For this review, take the finished solid that the model builds, in its own axes (mm). Round coordinates to 2 decimals unless told otherwise and drop trailing zeros. Order: outer loops, then holes, each group sorted by start corner. A loop starts at its lowest first (then second) coordinate and runs counter-clockwise, first axis right, second up.
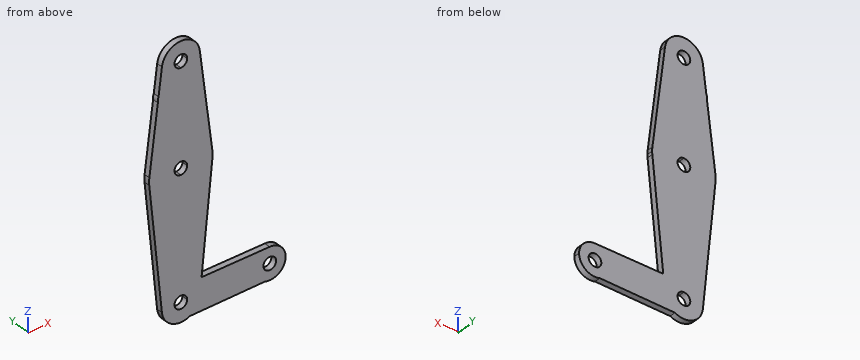
```python
from build123d import *

# Parameters (mm, degrees)
F1_DEPTH = 3.048


with BuildPart() as f1:
    # F0 (on Front) → F1 (new body)
    with BuildSketch(Plane.XZ):
        with BuildLine():
            ThreePointArc((-9.4502929642, 115.490625), (-7.14375, 107.9998046905), (0, 104.775))
            ThreePointArc((0, 104.775), (6.7351920908, 107.5648079092), (9.525, 114.3))
            ThreePointArc((9.525, 114.3), (9.5063048942, 114.896483242), (9.4502929642, 115.490625))
            ThreePointArc((9.4502929642, 115.490625), (0, 123.825), (-9.4502929642, 115.490625))
        make_face()
        with BuildLine():
            ThreePointArc((3.175, 114.3), (2.2450640303, 112.0549359697), (0, 111.125))
            ThreePointArc((0, 111.125), (-2.2450640303, 116.5450640303), (3.175, 114.3))
        make_face(mode=Mode.SUBTRACT)
        with BuildLine():
            ThreePointArc((9.525, 114.3), (6.7351920908, 107.5648079092), (0, 104.775))
            Line((0, 104.775), (0, 79.375))
            ThreePointArc((0, 79.375), (10.5003255158, 75.40625), (15.7504882737, 65.484375))
            Line((15.7504882737, 65.484375), (9.4502929642, 115.490625))
            ThreePointArc((9.4502929642, 115.490625), (9.5063048942, 114.896483242), (9.525, 114.3))
        make_face()
        with BuildLine():
            Line((0, 79.375), (0, 104.775))
            ThreePointArc((0, 104.775), (-7.14375, 107.9998046905), (-9.4502929642, 115.490625))
            Line((-9.4502929642, 115.490625), (-11.1502544755, 101.9975988084))
            ThreePointArc((-11.1502544755, 101.9975988084), (-5.3447623517, 105.1165944415), (-1.1603179203, 100.0252))
            ThreePointArc((-1.1603179203, 100.0252), (-5.9890709954, 94.8480839744), (-11.4894787169, 99.3050898642))
            Line((-11.4894787169, 99.3050898642), (-15.7504882737, 65.484375))
            ThreePointArc((-15.7504882737, 65.484375), (-10.5003255158, 75.40625), (0, 79.375))
        make_face()
        with BuildLine():
            ThreePointArc((15.7504882737, 65.484375), (10.5003255158, 75.40625), (0, 79.375))
            Line((0, 79.375), (0, 66.675))
            ThreePointArc((0, 66.675), (2.2450640303, 65.7450640303), (3.175, 63.5))
            ThreePointArc((3.175, 63.5), (2.2450640303, 61.2549359697), (0, 60.325))
            Line((0, 60.325), (0, 47.625))
            ThreePointArc((0, 47.625), (10.6492737428, 51.7267849017), (15.7954255641, 61.9125))
            ThreePointArc((15.7954255641, 61.9125), (15.8550939106, 62.7052534459), (15.875, 63.5))
            ThreePointArc((15.875, 63.5), (15.8438414904, 64.4941387366), (15.7504882737, 65.484375))
        make_face()
        with BuildLine():
            Line((0, 66.675), (0, 79.375))
            ThreePointArc((0, 79.375), (-10.5003255158, 75.40625), (-15.7504882737, 65.484375))
            ThreePointArc((-15.7504882737, 65.484375), (-15.8737438155, 63.6997054867), (-15.7954255641, 61.9125))
            ThreePointArc((-15.7954255641, 61.9125), (-10.6492737428, 51.7267849017), (0, 47.625))
            Line((0, 47.625), (0, 60.325))
            ThreePointArc((0, 60.325), (-3.175, 63.5), (0, 66.675))
        make_face()
        with BuildLine():
            ThreePointArc((-1.1603179203, 100.0252), (-5.3447623517, 105.1165944415), (-11.1502544755, 101.9975988084))
            Line((-11.1502544755, 101.9975988084), (-11.4894787169, 99.3050898642))
            ThreePointArc((-11.4894787169, 99.3050898642), (-5.9890709954, 94.8480839744), (-1.1603179203, 100.0252))
        make_face()
        with BuildLine():
            Line((-11.4894787169, 99.3050898642), (-11.1502544755, 101.9975988084))
            ThreePointArc((-11.1502544755, 101.9975988084), (-11.4989780624, 100.67391026), (-11.4894787169, 99.3050898642))
        make_face()
        with BuildLine():
            ThreePointArc((0, 47.625), (-10.6492737428, 51.7267849017), (-15.7954255641, 61.9125))
            Line((-15.7954255641, 61.9125), (-9.4772553384, -0.9525))
            ThreePointArc((-9.4772553384, -0.9525), (-7.063929059, 6.3895642457), (0, 9.525))
            Line((0, 9.525), (0, 47.625))
        make_face()
        with BuildLine():
            ThreePointArc((15.7954255641, 61.9125), (10.6492737428, 51.7267849017), (0, 47.625))
            Line((0, 47.625), (0, 9.525))
            ThreePointArc((0, 9.525), (3.0618336501, 9.0194678168), (5.7986582819, 7.5565327452))
            Line((5.7986582819, 7.5565327452), (10.336945567, 7.6013097722))
            Line((10.336945567, 7.6013097722), (15.7954255641, 61.9125))
        make_face()
        with BuildLine():
            ThreePointArc((0, 9.525), (-7.063929059, 6.3895642457), (-9.4772553384, -0.9525))
            ThreePointArc((-9.4772553384, -0.9525), (-4.4927588218, -8.3988536818), (4.4678891991, -8.4121097891))
            ThreePointArc((4.4678891991, -8.4121097891), (7.9074780174, -5.3101239538), (9.4772553384, -0.9525))
            ThreePointArc((9.4772553384, -0.9525), (9.5130563464, -0.4768479324), (9.525, 0))
            Line((9.525, 0), (3.175, 0))
            ThreePointArc((3.175, 0), (-2.2450640303, -2.2450640303), (0, 3.175))
            Line((0, 3.175), (0, 9.525))
        make_face()
        with BuildLine():
            Line((44.3716884408, 7.9371136788), (10.336945567, 7.6013097722))
            Line((10.336945567, 7.6013097722), (9.5729851903, 0))
            Line((9.5729851903, 0), (36.5125, 0))
            ThreePointArc((36.5125, 0), (38.8097205632, 5.5849041285), (44.3716884408, 7.9371136788))
        make_face()
        with BuildLine():
            Line((9.5729851903, 0), (10.336945567, 7.6013097722))
            Line((10.336945567, 7.6013097722), (5.7986582819, 7.5565327452))
            ThreePointArc((5.7986582819, 7.5565327452), (8.5427701928, 4.2126835191), (9.525, 0))
            Line((9.525, 0), (9.5729851903, 0))
        make_face()
        with BuildLine():
            ThreePointArc((9.4772553384, -0.9525), (7.9074780174, -5.3101239538), (4.4678891991, -8.4121097891))
            Line((4.4678891991, -8.4121097891), (42.0198443673, -7.5563383891))
            ThreePointArc((42.0198443673, -7.5563383891), (38.0354358455, -4.6751762488), (36.5125, 0))
            Line((36.5125, 0), (9.5729851903, 0))
            Line((9.5729851903, 0), (9.4772553384, -0.9525))
        make_face()
        with BuildLine():
            ThreePointArc((52.3875, 0), (50.0349041285, 5.6402794368), (44.3716884408, 7.9371136788))
            ThreePointArc((44.3716884408, 7.9371136788), (38.8097205632, 5.5849041285), (36.5125, 0))
            ThreePointArc((36.5125, 0), (38.0354358455, -4.6751762488), (42.0198443673, -7.5563383891))
            ThreePointArc((42.0198443673, -7.5563383891), (49.1251762488, -6.4145641545), (52.3875, 0))
        make_face()
        with BuildLine():
            ThreePointArc((47.625, 0), (44.45, -3.175), (41.275, 0))
            ThreePointArc((41.275, 0), (44.45, 3.175), (47.625, 0))
        make_face(mode=Mode.SUBTRACT)
        with BuildLine():
            ThreePointArc((5.7986582819, 7.5565327452), (3.0618336501, 9.0194678168), (0, 9.525))
            Line((0, 9.525), (0, 3.175))
            ThreePointArc((0, 3.175), (2.2450640303, 2.2450640303), (3.175, 0))
            Line((3.175, 0), (9.525, 0))
            ThreePointArc((9.525, 0), (8.5427701928, 4.2126835191), (5.7986582819, 7.5565327452))
        make_face()
    extrude(amount=F1_DEPTH)


solid = f1.part
```
Q1. Take a section at B-B, the plane x = 12. State the section outline as (y, z) points, plus the area to 3 significant figures.
Q2. Take a section at D-D, the plane x = 30. State the section outline as (y, z) points, plus the area to 3 significant figures.
Q3. Take a section at A-A, the plane y = -0.85. Count the separate pieces of the cut face and the enclosed holes in it, plus the area to 3 significant figures.
Q4. Take a section at C-C, the plane z = 23. State the section outline as (x, y) points.
Q5. Clearance check with flat-ended pins moving along their axes: pin 1 (1 mm diameter, centred on y = -1, z = 69.5, fed in from +X); pin 2 (1 mm diameter, centred on y = -0.5, z = 87.5, fed in from +X); pin 3 (1 mm diameter, centred on y = -1.5, z = 79, fed in from +X). State where each tip first meets the part, or that it passes through.
Q6. Wall thickness on line 1 (Z direction, x = 0, y = -0.85) (3 decimals); line 2 (X direction, y = -0.55, z = -1); line 3 (X direction, y = -0.85, z = 114.3) (3 decimals): over which ranges is each line inside the solid? List them lowest first.
Working result:
1. outline: (-3.05, -8.24) - (0, -8.24) - (0, 7.62) - (-3.05, 7.62) - close; (-3.05, 24.15) - (0, 24.15) - (0, 95.25) - (-3.05, 95.25) - close
1. area: 265 mm2
2. outline: (-3.05, -7.83) - (0, -7.83) - (0, 7.8) - (-3.05, 7.8) - close
2. area: 47.6 mm2
3. separate pieces: 1
3. enclosed holes: 5
3. area: 3,740 mm2
4. outline: (-11.88, -3.05) - (11.88, -3.05) - (11.88, 0) - (-11.88, 0) - close
5. pin 1: stops at x = 15.31
5. pin 2: stops at x = 13.04
5. pin 3: stops at x = 14.11
6. line 1: z = -9.525 to -3.175, 3.175 to 60.325, 66.675 to 111.125, 117.475 to 123.825
6. line 2: x = -9.47 to -3.01, 3.01 to 41.44, 47.46 to 52.32
6. line 3: x = -9.6 to -3.175, 3.175 to 9.6
